The model under review builds one solid part; all positions refer to its coordinate system, in mm. A direction names the side the tool comes from. Round coordinates to 2 decimals unless told otherwise and drop trailing zeros. Write each loop counter-clockwise with the first axis right and the second up, starting at its lowest first coordinate (ties: lowest second). Pieces come first, ordered by that corner, then holes. Notation, with made-up numbers: (15, -37.5) -> (73, -37.5) arc R11 cw to (73, -22.5) -> close; hole circle Ø2 at (-4.75, 30.5). An arc over 180 degrees is marked (long way). Answer in a Markdown table with one row per item. Add a question column.
```python
from build123d import *

# Parameters (mm, degrees)
SKETCH_W     = 60
SKETCH_H     = 60
SKETCH_W_2   = 54
SKETCH_H_2   = 54
PAD_DEPTH    = 610
SKETCH001_R  = 4.25
POCKET_DEPTH = 3
FILLET_R     = 3


with BuildPart() as part:
    # Sketch → Pad (new body)
    with BuildSketch(Plane.XZ):
        Rectangle(SKETCH_W, SKETCH_H)
        Rectangle(SKETCH_W_2, SKETCH_H_2, mode=Mode.SUBTRACT)
    extrude(amount=PAD_DEPTH)

    # Sketch001 (on Face1 of Pad) → Pocket (cut)
    with BuildSketch(Plane(origin=(0, 0, 30), x_dir=(-1, 0, 0), z_dir=(0, 0, 1))):
        with Locations((0, 30)):
            Circle(SKETCH001_R)
        with Locations((0, 580)):
            Circle(SKETCH001_R)
    extrude(amount=-POCKET_DEPTH, mode=Mode.SUBTRACT)

    # Fillet
    fillet_edges = [part.edges().sort_by_distance(p)[0] for p in [
        (30, -305, 30),
        (30, -305, -30),
        (-30, -305, 30),
        (-30, -305, -30),
    ]]
    fillet(fillet_edges, radius=FILLET_R)


solid = part.part
```
1. Add section B-B on z = 10. Write out the cut boundary in (x, y), plus the area to 3 significant figures.
2. For L1, parallel to Y at x = 0, z = 28; L2, parallel to Z at x = -25, y = -215, list the stretches that pass through material, from the lowest coordinate up.
3. Mouldability with a two-part tool opening along X and no side actions: class faces 1 (the flat face through (27, -301, 0)), 2 (the flat face through (-27, -301, 0)), 3 (the flat face through (-30, -301, 0)), 4 (the flat face through (30, -301, 0)) as pulls with the +X half, pulls with the -X half, needs draft (parallel to the pull), parting line crosses it, or undercut.
4. Add section C-C on y = -273. Write out the cut boundary in (x, z).
5. Add section A-A on x = -11. Write out the cut boundary in (y, z).
6. Tool access review of faces 5 (the flat face through (0, -301, 27)), 6 (the flat face through (0, -301, -30)): name each direction out of +Z, -Z, +X, -X, +Y, -Y from which nothing blocks a thin tool from reaching the whole face with its end or side.
Filled in:
| question | item | result |
|---|---|---|
| 1 | outline | (-30, -610) -> (-27, -610) -> (-27, 0) -> (-30, 0) -> close; (27, -610) -> (30, -610) -> (30, 0) -> (27, 0) -> close |
| 1 | area | 3,660 mm² |
| 2 | L1 | -610 to -584.25, -575.75 to -34.25, -25.75 to 0 |
| 2 | L2 | -30 to -27, 27 to 30 |
| 3 | face 1 | undercut |
| 3 | face 2 | undercut |
| 3 | face 3 | pulls with the -X half |
| 3 | face 4 | pulls with the +X half |
| 4 | outline | (-30, -27) arc R3 ccw to (-27, -30) -> (27, -30) arc R3 ccw to (30, -27) -> (30, 27) arc R3 ccw to (27, 30) -> (-27, 30) arc R3 ccw to (-30, 27) -> close; hole (-27, -27) -> (27, -27) -> (27, 27) -> (-27, 27) -> close |
| 5 | outline | (-610, -30) -> (0, -30) -> (0, -27) -> (-610, -27) -> close; (-610, 27) -> (0, 27) -> (0, 30) -> (-610, 30) -> close |
| 6 | face 5 | +Y, -Y |
| 6 | face 6 | -Z, +X, -X, +Y, -Y |
